The listing builds one solid part. Answer for the finished solid, in the listing's coordinates (mm). A direction names the side the tool comes from. Coordinates: 2 decimals unless noted, no trailing zeros. Write each loop counter-clockwise with the first axis right and the second up, starting at its lowest first coordinate (ties: lowest second). Pieces come first, ordered by that corner, then holes.
Autodesk Inventor part; units mm, degrees
ref_plane "YZ Plane" through (0, 0, 0) normal (1, 0, 0) x (0, 1, 0)
ref_plane "XZ Plane" through (0, 0, 0) normal (0, 1, 0) x (-1, 0, 0)
ref_plane "XY Plane" through (0, 0, 0) normal (0, 0, 1) x (1, 0, 0)
sketch "Náčrt1" plane through (0, 0, 0) normal (0, 1, 0) x (-1, 0, 0)
  circle A0 centre (0, 0) radius 16.5
  circle A1 centre (0, 0) radius 13.5
  dimension "d0" = 33
  dimension "d1" = 27
extrude "Vysunutí1" add sketch "Náčrt1" along normal mid plane 25 contours A1
sketch "Náčrt4" plane through (0, 0, 0) normal (1, 0, 0) x (0, 1, 0)
  line L0 (-12.5, 13.5) -> (-12.5, -13.5)
  point P0 (0, 0)
  point P1 (-8.5, 0)
  dimension "d16" = 4
hole "Díra2" at (0, -8.5, 0) direction (1, 0, 0) diameter 3 end through all
thread "Závit1"
extrude "Vysunutí2" add sketch "Náčrt1" along normal mid plane 22
sketch "Náčrt2" plane through (0, 12.5, 0) normal (0, 1, 0) x (1, 0, 0)
  circle A0 centre (0, 0) radius 9
  dimension "d6" = 18
extrude "Vysunutí3" cut sketch "Náčrt2" against normal blind 14.5
sketch "Náčrt3" plane through (0, -12.5, 0) normal (0, -1, 0) x (1, 0, 0)
  circle A0 centre (0, 0) radius 13.5
hole "Díra1" at (0, -12.5, 0) direction (0, 1, 0) diameter 3 end through all
properties part number "JSUMO_Wheel_33x20mm"
Q1. Which of the six approach directions +Z, -Z, +X, -X, +Y, -Y give full straight-line access (tool end or side, diameter ignored) to faces 1 (the face through (13.5, -8.5, 0)), 2 (the face through (-3, -12.5, 0)), 3 (the face through (14, -11, 0)), 4 (the face through (-1.487, -7.176, 0.195)), 5 (the face through (14, 11, 0))?
Answers below:
face 1: none
face 2: +Z, -Z, +X, -X, -Y
face 3: -Y
face 4: +Y, -Y
face 5: +Y
Q2. Given pin 1 (1.8 mm diameter, centred on x = 0, z = 0, fed in from +Y); pin 2 (9 mm diameter, centred on x = 2, z = -2.5, fed in from +Y); pin 3 (12 mm diameter, centred on x = -7, y = 4.5, fed in from +Z); pin 4 (6 mm diameter, centred on x = 10.5, y = -6.5, fed in from +Z), each flat-ended and moving along its own axis, determine where each tip first touches the part or whether it passes through.
Answers below:
pin 1: passes through
pin 2: stops at y = -2
pin 3: stops at z = 16.47
pin 4: stops at z = 14.7
Q3. The part is cut by section A-A, the plane z = 0. Write down the section's boundary in (x, y), then the cut area to 4 significant figures.
Answers below:
outline: (-16.5, -11) - (-13.5, -11) - (-13.5, -12.5) - (-1.5, -12.5) - (-1.5, -2) - (-9, -2) - (-9, 12.5) - (-13.5, 12.5) - (-13.5, 11) - (-16.5, 11) - close; (1.5, -12.5) - (13.5, -12.5) - (13.5, -11) - (16.5, -11) - (16.5, 11) - (13.5, 11) - (13.5, 12.5) - (9, 12.5) - (9, -2) - (1.5, -2) - (1.5, -7) - (13.5, -7) - (13.5, -10) - (1.5, -10) - close
area: 478.5 mm2
Q4. The part is cut by section C-C, the plane y = -8.5. Write down the section's boundary in (x, z).
Answers below:
outline: circle Ø33 at (0, 0); hole (0, -1.5) - (13.42, -1.5) arc R13.5 ccw to (13.42, 1.5) - (0, 1.5) arc R1.5 ccw to start
Q5. Find the intervals of material crossed by probe 1 along Z at (x, y) = (0, -4.5); probe 2 along Y at (x, z) = (8, 0); probe 3 along Z at (x, y) = (-2, -1.5), in increasing order.
Answers below:
probe 1: z = -16.5 to -1.5, 1.5 to 16.5
probe 2: y = -12.5 to -10, -7 to -2
probe 3: z = -16.38 to -8.77, 8.77 to 16.38
Q6. Determine the mould class of faces 6 (the face through (2.93, -11.76, 13.18)), 7 (the face through (6.845, -7.925, 1.386)), 8 (the face through (-9, 12.5, -3)) for opening direction Z: released by +Z, released by -Z, zero draft, split by the parting line, or undercut.
Answers below:
face 6: split by the parting line
face 7: undercut
face 8: zero draft
Q7. The part is cut by section B-B, the plane x = 9.5. Write down the section's boundary in (y, z).
Answers below:
outline: (-12.5, -9.59) - (-11, -9.59) - (-11, -13.49) - (11, -13.49) - (11, -9.59) - (12.5, -9.59) - (12.5, 9.59) - (11, 9.59) - (11, 13.49) - (-11, 13.49) - (-11, 9.59) - (-12.5, 9.59) - close; hole circle Ø3 at (-8.5, 0)
Q8. The part is cut by section D-D, the plane x = -2. Write down the section's boundary in (y, z), then the cut area to 3 significant figures.
Answers below:
outline: (-12.5, -13.35) - (-11, -13.35) - (-11, -16.38) - (11, -16.38) - (11, -13.35) - (12.5, -13.35) - (12.5, -8.77) - (-2, -8.77) - (-2, 8.77) - (12.5, 8.77) - (12.5, 13.35) - (11, 13.35) - (11, 16.38) - (-11, 16.38) - (-11, 13.35) - (-12.5, 13.35) - close
area: 546 mm2
